from build123d import *

# Parameters (mm, degrees)
EXTRUDE_1_DEPTH     = 13
SKETCH_5_R          = 7.5
CUT_EXTRUDE_1_DEPTH = 23.472205054
CHAMFER_1_SIZE      = 0.5


with BuildPart() as part:
    # Эскиз1 → Вытянуть1 (new body)
    with BuildSketch(Plane(origin=(0, 0, 0), x_dir=(1, 0, 0), z_dir=(0, 1, 0))):
        Polygon((-6.92820323, 12), (6.92820323, 12), (13.856406461, 0), (6.92820323, -12), (-6.92820323, -12), (-13.856406461, 0), align=None)
    extrude(amount=-EXTRUDE_1_DEPTH)

    # Эскиз5 → Вырез-Вытянуть1 (cut, through all)
    with BuildSketch(Plane.XZ.offset(13)):
        with Locations(Location((0, 0, 0), (0, 0, 270))):
            Circle(SKETCH_5_R)
    extrude(amount=-CUT_EXTRUDE_1_DEPTH, mode=Mode.SUBTRACT)

    # Эскиз4 → Вырез-Повернуть1 (revolve, cut)
    with BuildSketch(Plane.XY, mode=Mode.PRIVATE) as cut_revolve_1_sk:
        Polygon((-13.856406461, -1.649147039), (-11, 0), (-13.856406461, 0), align=None)
        Polygon((-13.856406461, -11.350852961), (-11, -13), (-13.856406461, -13), align=None)
    revolve(cut_revolve_1_sk.sketch.rotate(Axis((0, 0, 0), (0, -1, 0)), 119.999999992), axis=Axis((0, 0, 0), (0, -1, 0)), mode=Mode.SUBTRACT)

    # Фаска1
    chamfer_1_edges = [part.edges().sort_by_distance(p)[0] for p in [
        (0, 0, 7.5),
        (0, -13, 7.5),
    ]]
    chamfer(chamfer_1_edges, length=CHAMFER_1_SIZE)


solid = part.part
The model under review builds one solid part; all positions refer to its coordinate system, in mm. Coordinates: 2 decimals unless noted, no trailing zeros. Loops run counter-clockwise (first coordinate to the right, second up) from the corner with the lowest first, then second, coordinate; pieces in that order, holes last. Notation, with made-up numbers: M -28,24.25 L 31,24.25 A20 cw 31,44.25 Z; hole C 88.5,16 d9. An arc over 180 degrees is marked long. Put each result on its own line as item: value. Start each with the question number.
Q1. The part is to be moulded in two halves that separate along X. For faces 1 (the cylindrical face through (0.33, -6.584, 7.493)), 2 (the flat face through (10.44, -6.42, 5.92)), 3 (the flat face through (-10.44, -6.42, -5.92)), say which applies: +X half, -X half, draft (parallel to the pull), parting line (faces both ways), or undercut.
Q2. Add section A-A (x = 0). Write out the cut boundary in (y, z).
Q3. Wall thickness on line 1 (X direction, y = -11.75, z = -4); line 2 (X direction, y = -12.25, z = 0.5); line 3 (Z direction, x = -10, y = -3.75): over which ranges is each line inside the solid? List them lowest first.
Q4. Add section B-B (y = -2). Write out the cut boundary in (x, z), and give its area (3 significant figures).
Q5. Clearance check with a flat-ended pin moving along its axis: pin 1 (13.5 mm diameter, centred on x = 0, z = 0, fed in from -Y). State where the tip first meets the part, or that it passes through.
Answers:
1. face 1: undercut
1. face 2: +X half
1. face 3: -X half
2. outline: M -13,-11 L -12.42,-12 L -0.58,-12 L 0,-11 L 0,-8 L -0.5,-7.5 L -12.5,-7.5 L -13,-8 Z; M -13,8 L -12.5,7.5 L -0.5,7.5 L 0,8 L 0,11 L -0.58,12 L -12.42,12 L -13,11 Z
3. line 1: x = -11.55 to -6.34, 6.34 to 11.55
3. line 2: x = -12.29 to -7.48, 7.48 to 12.29
3. line 3: z = -6.68 to 6.68
4. outline: M -13.86,0 L -6.93,-12 L 6.93,-12 L 13.86,0 L 6.93,12 L -6.93,12 Z; hole C 0,0 d15
4. area: 322 mm^2
5. pin 1: passes through
